```python
from build123d import *

# Parameters (mm, degrees)
F0_R     = 24.13
F1_DEPTH = 228.6
F2_R     = 6.35
F3_DEPTH = 66.294
F4_W     = 79.389766
F4_H     = 50.704014
F5_DEPTH = 4.826


with BuildPart() as f1:
    # F0 (on Top) → F1 (new body)
    with BuildSketch(Plane.XY):
        with Locations((-7.287733, 25.4)):
            Circle(F0_R)
    extrude(amount=F1_DEPTH)

    # F2 (on Front) → F3 (cut)
    with BuildSketch(Plane.XZ):
        with Locations((-7.949968, 183.391028)):
            Circle(F2_R)
    extrude(amount=-F3_DEPTH, mode=Mode.SUBTRACT)

    # F4 (on Top) → F5 (join)
    with BuildSketch(Plane.XY):
        with Locations((-6.667502, 25.352007)):
            Rectangle(F4_W, F4_H)
    extrude(amount=F5_DEPTH)


solid = f1.part
```
Part model, mm, in its own coordinate system. Round coordinates to 2 decimals unless told otherwise and drop trailing zeros. Write each loop counter-clockwise with the first axis right and the second up, starting at its lowest first coordinate (ties: lowest second). Pieces come first, ordered by that corner, then holes. Notation, with made-up numbers: M -30,76.25 L 24,76.25 A4 cw 24,82.25 Z; hole C -33,56 d3. An arc over 180 degrees is marked long. Answer as CSV lines item,"result". Start each with the question number.
1) Band-saw the part on A-A (y = 21). List the corners of the cut face in (x, z), then the cut area to 3 significant figures.
2) Band-saw the part on B-B (z = 60). List the corners of the cut face in (x, y).
3) Mould opens along Z. For faces 1 (the face through (-12.519, 1.844, 115.147)), 2 (the face through (-8.777, 25.062, 189.687)), 3 (the face through (2, 48, 4.826)) say: +Z half, -Z half, draft (parallel to the pull), parting line (faces both ways), or undercut.
4) Drop flat-ended pins along their axis: pin 1 (3 mm diameter, centred on x = 1.5, z = 141.5, fed in from +Y); pin 2 (1 mm diameter, centred on y = 36, z = 59, fed in from +X); pin 3 (6 mm diameter, centred on x = -36, y = 36.5, fed in from +Z); pin 4 (10 mm diameter, centred on x = -26.5, y = 9.5, fed in from +Z). Give the stop position or say it passes through.
5) Drill centre lines: L1, parallel to Z at x = -36, y = 22; L2, parallel to Y at x = -8, z = 12; L3, parallel to Z at x = -10, y = 47.5. Where is each one in solid material? Low to high.
6) Band-saw the part on C-C (y = 46). List the corners of the cut face in (x, z), then the cut area to 3 significant figures.
Worked out:
1,outline,"M -46.36,0 L 33.03,0 L 33.03,4.83 L 16.44,4.83 L 16.44,228.6 L -31.01,228.6 L -31.01,4.83 L -46.36,4.83 Z; hole C -7.95,183.39 d12.7"
1,area,"10,900 mm²"
2,outline,"C -7.29,25.4 d48.26"
3,face 1,"draft"
3,face 2,"undercut"
3,face 3,"+Z half"
4,pin 1,"y = 48.4"
4,pin 2,"x = 14.63"
4,pin 3,"z = 4.83"
4,pin 4,"z = 228.6"
5,L1,"0 to 4.83"
5,L2,"1.28 to 49.52"
5,L3,"0 to 177.38, 189.4 to 228.6"
6,outline,"M -46.36,0 L 33.03,0 L 33.03,4.83 L 5.28,4.83 L 5.28,228.6 L -19.85,228.6 L -19.85,4.83 L -46.36,4.83 Z; hole C -7.95,183.39 d12.7"
6,area,"5,880 mm²"
